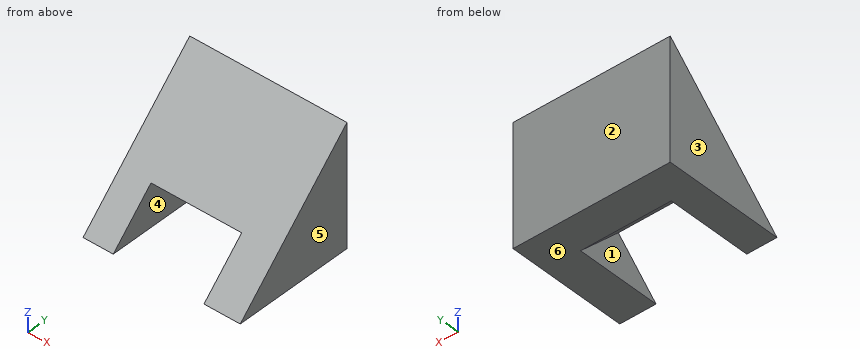
```python
from build123d import *

# Parameters (mm, degrees)
F0_W     = 33.02
F0_H     = 25.4
F1_DEPTH = 12.7
F3_DEPTH = 33.021
F4_W     = 19.05
F4_H     = 12.7
F5_DEPTH = 12.7


with BuildPart() as f1:
    # F0 (on Front) → F1 (new body, symmetric)
    with BuildSketch(Plane.XZ):
        with Locations((16.51, 12.7)):
            Rectangle(F0_W, F0_H)
    extrude(amount=F1_DEPTH, both=True)

    # F2 (on face) → F3 (cut, through all)
    with BuildSketch(Plane.YZ.offset(33.02)):
        Polygon((-12.7, 0), (12.7, 25.4), (-12.7, 25.4), align=None)
    extrude(amount=-F3_DEPTH, mode=Mode.SUBTRACT)

    # F4 (on face) → F5 (cut)
    with BuildSketch(Plane(origin=(0, -6.35, 6.35), x_dir=(1, 0, 0), z_dir=(0, -0.707107, 0.707107))):
        with Locations((15.875, -2.630256)):
            Rectangle(F4_W, F4_H)
    extrude(amount=-F5_DEPTH, mode=Mode.SUBTRACT)


solid = f1.part
```
Could you check a few things on this model? Use its own coordinates, in mm. Face numbers are marked on the shaded views. A direction names the side the tool comes from. Round coordinates to 2 decimals unless told otherwise and drop trailing zeros. Order: outer loops, then holes, each group sorted by start corner. A loop starts at its lowest first (then second) coordinate and runs counter-clockwise, first axis right, second up. Notation, with made-up numbers: M 74.5,71.25 L 93.5,71.25 A31 cw 93.5,106.25 Z; hole C 68.5,88 d1. An arc over 180 degrees is marked long. One line per question, with ' | ' between items. Start each with the question number.
(1) Suppose I cut it at B-B on y = -8.75. List the corners of the cut face in (x, z) for me.
(2) Suppose I cut it at A-A on y = -4.75. List the corners of the cut face in (x, z) for me, then the cut area to 3 significant figures.
(3) Thinking about a two-plate mould opening in X: for the marked faces 3, 4, 5 and 6, which applies, +X half, -X half, draft (parallel to the pull), parting line (faces both ways), or undercut?
(4) Please list where these lines run through material, in increasing order: line 1 along Y through (x, z) = (3.5, 20); line 2 along Z through (x, y) = (26, 10); line 3 along Y through (x, z) = (2, 16.5).
(5) For P1, Ø2, axis at y = -9, z = 7.5, coming from the -X side; P2, Ø1, axis at x = 7.5, y = 5.5, coming from the +Z side; P3, Ø12, axis at x = 16, y = -3, coming from the -Z side; P4, Ø4, axis at x = 25, y = -3.5, coming from the +Z side, each with a flat end and sliding along its axis, tell me the tip position at first contact or that it passes through.
(6) For the marked faces 1 and 2, which set-ups out of +Z, -Z, +X, -X, +Y, -Y let a thin tool reach every point of the face, with its end or its side?
(7) Suppose I cut it at D-D on x = 17. List the corners of the cut face in (y, z) for me.
(8) Suppose I cut it at C-C on z = 5. List the corners of the cut face in (x, y) for me.
Geometry results:
1) outline: M 0,0 L 6.35,0 L 6.35,3.95 L 0,3.95 Z; M 25.4,0 L 33.02,0 L 33.02,3.95 L 25.4,3.95 Z
2) outline: M 0,0 L 6.35,0 L 6.35,7.95 L 0,7.95 Z; M 25.4,0 L 33.02,0 L 33.02,7.95 L 25.4,7.95 Z | area: 111 mm²
3) face 3: -X half | face 4: undercut | face 5: +X half | face 6: draft
4) line 1: 7.3 to 12.7 | line 2: 0 to 22.7 | line 3: 3.8 to 12.7
5) P1: through | P2: z = 18.7 | P3: z = 2.26 | P4: z = 11.2
6) face 1: -Z, -Y | face 2: +Z, -Z, +X, -X, +Y
7) outline: M -3.72,8.98 L 5.26,0 L 12.7,0 L 12.7,25.4 Z
8) outline: M 0,-7.7 L 6.35,-7.7 L 6.35,0.26 L 25.4,0.26 L 25.4,-7.7 L 33.02,-7.7 L 33.02,12.7 L 0,12.7 Z
